```python
from build123d import *


with BuildPart() as part:
    # Sketch2 → Revolve1 (revolve)
    with BuildSketch(Plane.XY):
        with BuildLine():
            Line((0, 0), (0, 220))
            Line((0, 220), (20, 220))
            ThreePointArc((20, 220), (30, 210), (20, 200))
            Line((20, 200), (20, 160))
            ThreePointArc((20, 160), (40, 140), (20, 120))
            Line((20, 120), (20, 80))
            ThreePointArc((20, 80), (37.573593129, 37.573593129), (80, 20))
            ThreePointArc((80, 20), (91.180339887, 13.090169944), (90, 0))
            Line((90, 0), (0, 0))
        make_face()
    revolve(axis=Axis((0, 0, 0), (0, 1, 0)))


solid = part.part
```
Can you work these out from the model? Positions are in its coordinate system, mm. Coordinates: 2 decimals unless noted, no trailing zeros. Put each result on its own line as item: value. Start each with the question number.
(1) I need wall thicknesses on probe 1 along Y at (x, z) = (76, -21.5); probe 2 along Z at (x, y) = (4, 115); probe 3 along Y at (x, z) = (-85, 19.5). Which ranges of each line are inside material? Lowest first, please.
(2) Will this pin go through, and if not, where does the flat tip stop? pin 1 Ø6 at (x, y) = (20, 85.5) entering from +Z.
(3) We'd pull the mould along Y, two halves only. Please class faces 1 (the face through (-4.336, 179.72, 19.524)), 2 (the face through (0, 220, 0)), 3 (the face through (-1, 0, -1)): +Y half, -Y half, draft (parallel to the pull), parting line (faces both ways), or undercut.
Worked answers:
1. probe 1: y = 0 to 20.01
1. probe 2: z = -19.6 to 19.6
1. probe 3: y = 0 to 17.71
2. pin 1: stops at z = 10.54
3. face 1: undercut
3. face 2: +Y half
3. face 3: -Y half
